```python
from build123d import *

# Parameters (mm, degrees)
F0_W     = 990.6
F0_H     = 685.8
F1_DEPTH = 38.1
F2_R     = 6.35
F3_W     = 38.1
F3_H     = 152.4
F4_DEPTH = 38.1


with BuildPart() as f1:
    # F0 (on Top) → F1 (new body)
    with BuildSketch(Plane.XY):
        with Locations((495.3, 342.9)):
            Rectangle(F0_W, F0_H)
    extrude(amount=F1_DEPTH)

    # F2
    f2_edges = [f1.edges().sort_by_distance(p)[0] for p in [
        (0, 342.9, 38.1),
        (495.3, 0, 38.1),
        (990.6, 342.9, 38.1),
        (495.3, 685.8, 38.1),
        (0, 342.9, 0),
        (495.3, 0, 0),
        (990.6, 342.9, 0),
        (495.3, 685.8, 0),
        (0, 0, 19.05),
        (990.6, 0, 19.05),
        (990.6, 685.8, 19.05),
        (0, 685.8, 19.05),
    ]]
    fillet(f2_edges, radius=F2_R)

    # F3 (on face) → F4 (cut, through all)
    with BuildSketch(Plane.XY.offset(38.1)):
        with Locations((107.95, 342.9)):
            Rectangle(F3_W, F3_H)
        with Locations((882.65, 342.9)):
            Rectangle(F3_W, F3_H)
    extrude(amount=-F4_DEPTH, mode=Mode.SUBTRACT)


solid = f1.part
```
Geometry: final body of the model. Coordinates: model frame, mm. A direction names the side the tool comes from. Coordinates: 2 decimals unless noted, no trailing zeros. Order: outer loops, then holes, each group sorted by start corner. A loop starts at its lowest first (then second) coordinate and runs counter-clockwise, first axis right, second up. Notation, with made-up numbers: (28.25, 12.25) -> (55.25, 12.25) arc R30 cw to (55.25, 46.25) -> close; hole circle Ø5 at (46, -14.75). An arc over 180 degrees is marked (long way). Answer in a Markdown table with one row per item.
Item 1: Contact query for a flat-ended pin moving along its axis: P1, Ø1, axis at y = 559, z = 33.5, coming from the -X side. Output: stop coordinate, or through.
Return value:
| item | result |
|---|---|
| P1 | stops at x = 0.12 |
Item 2: Access query for faces 4 (the flat face through (488, 348, 38.1)), 5 (the flat face through (88.9, 342, 19)). Directions: +Z, -Z, +X, -X, +Y, -Y. A direction counts if a zero-diameter tool reaches every point of the face in a straight line with its end or side. Return the directions, or none.
Return value:
| item | result |
|---|---|
| face 4 | +Z, +X, -X, +Y, -Y |
| face 5 | +Z, -Z |
Item 3: Section B-B on z = 21. Output: boundary loops of the cut face in (x, y).
Return value:
| item | result |
|---|---|
| outline | (0, 6.35) arc R6.35 ccw to (6.35, 0) -> (984.25, 0) arc R6.35 ccw to (990.6, 6.35) -> (990.6, 679.45) arc R6.35 ccw to (984.25, 685.8) -> (6.35, 685.8) arc R6.35 ccw to (0, 679.45) -> close; hole (88.9, 266.7) -> (127, 266.7) -> (127, 419.1) -> (88.9, 419.1) -> close; hole (863.6, 266.7) -> (901.7, 266.7) -> (901.7, 419.1) -> (863.6, 419.1) -> close |
Item 4: Section A-A on y = 304. Output: boundary loops of the cut face in (x, z), plus the area to 3 significant figures.
Return value:
| item | result |
|---|---|
| outline | (0, 6.35) arc R6.35 ccw to (6.35, 0) -> (88.9, 0) -> (88.9, 38.1) -> (6.35, 38.1) arc R6.35 ccw to (0, 31.75) -> close; (127, 0) -> (863.6, 0) -> (863.6, 38.1) -> (127, 38.1) -> close; (901.7, 0) -> (984.25, 0) arc R6.35 ccw to (990.6, 6.35) -> (990.6, 31.75) arc R6.35 ccw to (984.25, 38.1) -> (901.7, 38.1) -> close |
| area | 34,800 mm² |
Item 5: Draft query along Y for faces 1 (the flat face through (882, 266.7, 19)), 2 (the flat face through (0, 338, 19)), 3 (the flat face through (488, 0, 19)). Return one class per face: released by +Y, released by -Y, zero draft, split by the parting line, or undercut.
Return value:
| item | result |
|---|---|
| face 1 | undercut |
| face 2 | zero draft |
| face 3 | released by -Y |
Item 6: Ray query, L1, parallel to X at y = 372, z = 6; L2, parallel to Y at x = 881, z = 24; L3, parallel to Y at x = 943, z = 33. Return the intervals inside material, ascending.
Return value:
| item | result |
|---|---|
| L1 | x = 0.01 to 88.9, 127 to 863.6, 901.7 to 990.59 |
| L2 | y = 0 to 266.7, 419.1 to 685.8 |
| L3 | y = 0.12 to 685.68 |
